Geometry: final body of the model. Coordinates: model frame, mm. Give positions to 0.01 mm unless a question says otherwise; leave off trailing zeros. Order: outer loops, then holes, each group sorted by start corner. A loop starts at its lowest first (then second) coordinate and runs counter-clockwise, first axis right, second up. Notation, with made-up numbers: (-18, 80) -> (8, 80) arc R26 cw to (8, 95) -> close; hole circle Ø9 at (48, 21.5). An arc over 180 degrees is marked (long way). One line per question, with ' | ' between items.
from build123d import *

# Parameters (mm, degrees)
F1_DEPTH = 19.05
F2_DEPTH = 19.05


with BuildPart() as f1:
    # F0 (on Top) → F1 (new body)
    with BuildSketch(Plane.XY):
        Polygon((-107.763073, 107.763073), (-287.368196, 107.763073), (107.763073, -287.368196), (107.763073, -107.763073), align=None)
    extrude(amount=F1_DEPTH)

    # F0 (on Top) → F2 (join)
    with BuildSketch(Plane.XY):
        Polygon((-107.763073, 287.368196), (-107.763073, 107.763073), (107.763073, -107.763073), (287.368196, -107.763073), align=None)
    extrude(amount=F2_DEPTH)


solid = f1.part
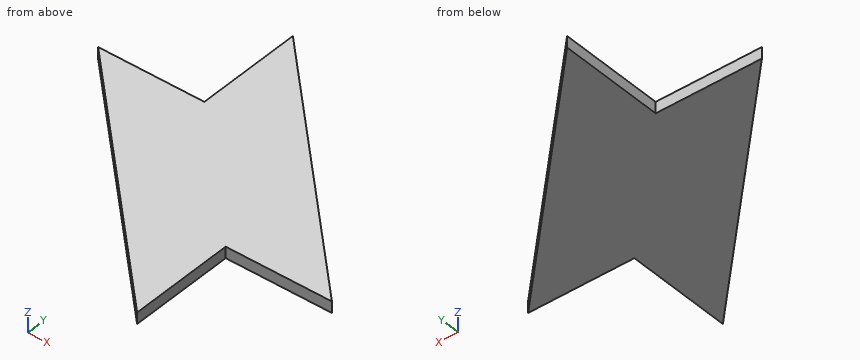
1) Material intervals for probe 1 along Y at (x, z) = (-123.5, 10); probe 2 along Y at (x, z) = (-93.5, 17.5); probe 3 along X at (y, z) = (138.5, 5.5), sorted ascending. Write a range as from..to.
Check result:
probe 1: y = -56.11..107.76 | probe 2: y = -86.11..273.11 | probe 3: x = -107.76..41.11
2) Section B-B on y = -184.5. Return loops of the section in (x, z).
Check result:
outline: (4.89, 0) -> (107.76, 0) -> (107.76, 19.05) -> (4.89, 19.05) -> close
3) Section A-A on z = 6.25. Return loops of the section in (x, y), plus the area to 3 significant figures.
Check result:
outline: (-287.37, 107.76) -> (107.76, -287.37) -> (107.76, -107.76) -> (287.37, -107.76) -> (-107.76, 287.37) -> (-107.76, 107.76) -> close | area: 110,000 mm^2
4) Contact query for flat-ended pins moving along their axis: pin 1 Ø3 at (x, z) = (-70, 11.5) entering from -Y; pin 2 Ø9.5 at (y, z) = (215.5, 8.5) entering from -X; pin 3 Ø5.5 at (x, z) = (-199, 9.5) entering from +Y. Output: stop coordinate, or through.
Check result:
pin 1: stops at y = -111.11 | pin 2: stops at x = -107.76 | pin 3: stops at y = 107.76
5) Section C-C on x = 158.5. Return loops of the section in (y, z), plus the area to 3 significant figures.
Check result:
outline: (-107.76, 0) -> (21.11, 0) -> (21.11, 19.05) -> (-107.76, 19.05) -> close | area: 2,450 mm^2
